Print and shaded views of the part. All mm, measured from the part's lowest x, y and z. A direction names the side the tool comes from. Coordinates: 2 decimals unless noted, no trailing zeros. Write each loop counter-clockwise with the first axis right and the second up, starting at its lowest first coordinate (ties: lowest second). Pieces come first, ordered by that corner, then holes. Notation, with made-up numbers: (50, -17.5) -> (83, -17.5) arc R17 cw to (83, -5.5) -> close; hole circle Ø6 at (-2, 72.25). An arc over 180 degrees is marked (long way). Write item = value, one per line.
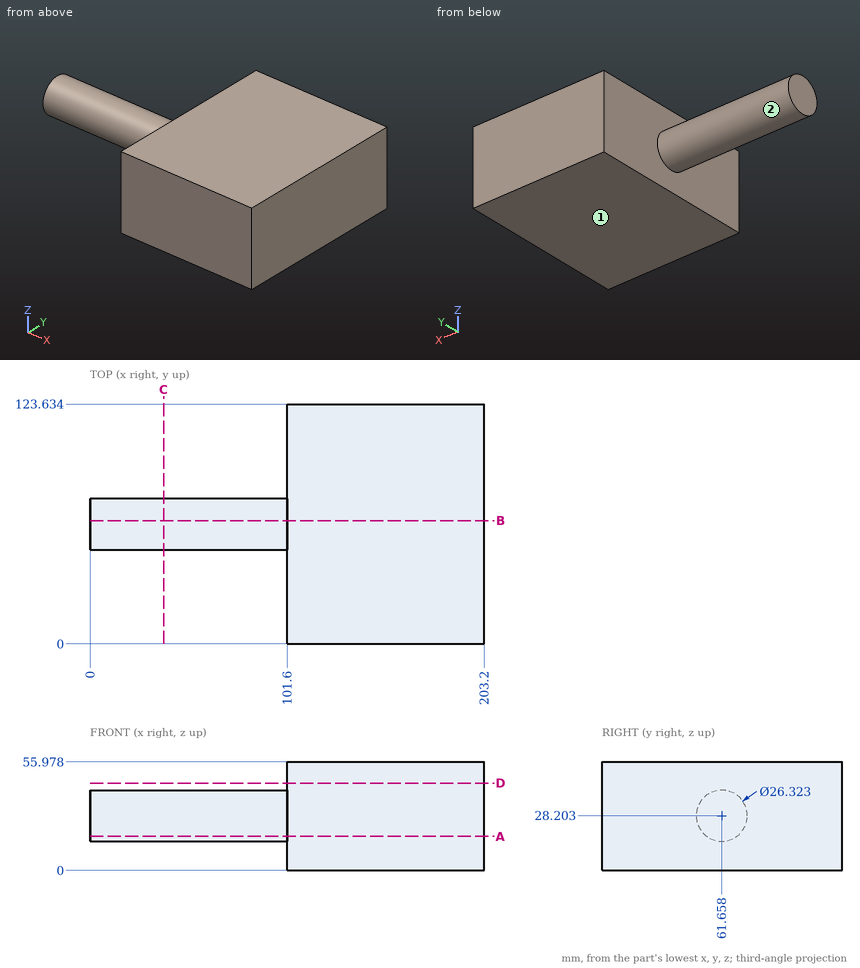
Q1. Which spindle directions (+Z, -Z, +X, -X, +Y, -Y) get a long thin tool onto all of the face, cutting with end or side? Do the marked faces 1 and 2. Say none if no direction does.
Model answer:
face_1 = -Z, +X, -X, +Y, -Y
face_2 = -X
Q2. Pin check, flat tips, straight feed: pin 1 (1.5 mm diameter, centred on y = 46.5, z = 31, fed in from -X); pin 2 (3 mm diameter, centred on x = 80.5, z = 43.5, fed in from -Y); pin 3 (10 mm diameter, centred on x = 169.5, y = 55.5, fed in from -Z); pin 4 (8 mm diameter, centred on x = 42, z = 41, fed in from +Y). Stop position of each tip, or through.
Model answer:
pin_1 = 101.6
pin_2 = through
pin_3 = 0
pin_4 = 71.45
Q3. Saw through at B-B on y = 63.5. Give the cut face in (x, z) (1 decimal).
Model answer:
outline = (0, 15.2) -> (101.6, 15.2) -> (101.6, 0) -> (203.2, 0) -> (203.2, 56) -> (101.6, 56) -> (101.6, 41.2) -> (0, 41.2) -> close
Q4. Saw through at A-A on z = 17.5. Give the cut face in (x, y), and give its area (3 significant figures).
Model answer:
outline = (0, 54) -> (101.6, 54) -> (101.6, 0) -> (203.2, 0) -> (203.2, 123.63) -> (101.6, 123.63) -> (101.6, 69.32) -> (0, 69.32) -> close
area = 14,100 mm²
Q5. Saw through at D-D on z = 45. Give the cut face in (x, y).
Model answer:
outline = (101.6, 0) -> (203.2, 0) -> (203.2, 123.63) -> (101.6, 123.63) -> close
Q6. Probe line 1 (X direction, y = 81.5, z = 23); line 2 (Z direction, x = 64, y = 64); line 3 (Y direction, x = 51, z = 22.5). List the from-to ranges inside material, lowest first. Write a range as from..to.
Model answer:
line_1 = 101.6..203.2
line_2 = 15.25..41.15
line_3 = 49.8..73.52
Q7. Saw through at C-C on x = 38. Give the cut face in (y, z).
Model answer:
outline = circle Ø26.32 at (61.66, 28.2)
